Can you work these out from the model? Positions are in its coordinate system, mm. Face numbers are marked on the shaded views. A direction names the side the tool comes from. Give positions to 0.01 mm unless a question says otherwise; leave off trailing zeros. Loops run counter-clockwise (first coordinate to the right, second up) from the corner with the lowest first, then second, coordinate; pieces in that order, holes last.
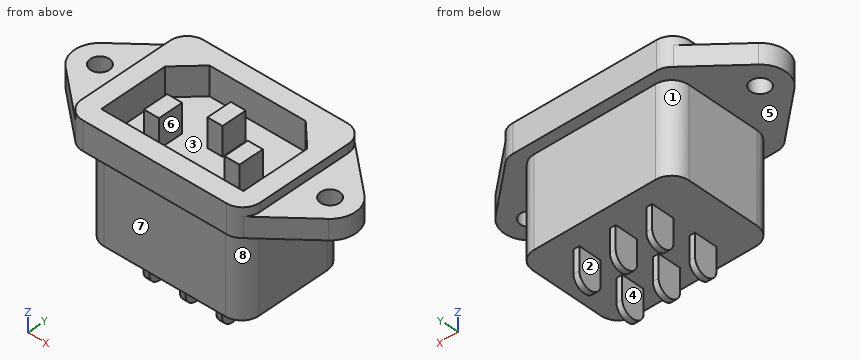
Autodesk Inventor part; units mm, degrees
ref_plane "YZ Plane" through (0, 0, 0) normal (1, 0, 0) x (0, 1, 0)
ref_plane "XZ Plane" through (0, 0, 0) normal (0, 1, 0) x (-1, 0, 0)
ref_plane "XY Plane" through (0, 0, 0) normal (0, 0, 1) x (1, 0, 0)
sketch "Base" plane through (0, 0, 0) normal (0, 0, 1) x (1, 0, 0)
  line L0 (-12.5, -11.25) -> (12.5, -11.25)
  line L1 (15.5, -8.25) -> (15.5, 8.25)
  line L2 (12.5, 11.25) -> (-12.5, 11.25)
  line L3 (-15.5, 8.25) -> (-15.5, -8.25)
  line L4 (-15.5, -11.25) -> (15.5, 11.25) construction
  line L5 (15.5, -11.25) -> (-15.5, 11.25) construction
  line L6 (-34.16, 0) -> (34.16, 0) construction
  line L7 (0, -16.6198) -> (0, 16.6198) construction
  circle A0 centre (-20, 0) radius 1.65
  circle A1 centre (20, 0) radius 1.65
  circle A2 centre (-20, 0) radius 4.4
  circle A3 centre (20, 0) radius 4.4
  line L8 (-24.4, 0) -> (24.4, 0) construction
  arc A4 (-12.5, 11.25) -> (-15.5, 8.25) centre (-12.5, 8.25) ccw
  arc A5 (-15.5, -8.25) -> (-12.5, -11.25) centre (-12.5, -8.25) ccw
  arc A6 (15.5, 8.25) -> (12.5, 11.25) centre (12.5, 8.25) ccw
  arc A7 (12.5, -11.25) -> (15.5, -8.25) centre (12.5, -8.25) ccw
  line L9 (-22.8555, 3.3476) -> (-14.6213, 10.3713)
  line L10 (14.6213, 10.3713) -> (22.8555, 3.3476)
  line L11 (-22.8555, -3.3476) -> (-14.6213, -10.3713)
  line L12 (14.6213, -10.3713) -> (22.8555, -3.3476)
  point P0 (0, 0)
  dimension "d0" = 31
  dimension "d1" = 22.5
  dimension "d2" = 3.3
  dimension "d3" = 48.8
  dimension "d4" = 40
  dimension "d15" = 3
  dimension "d16" = 3
extrude "BaseFeature" add sketch "Base" along normal blind 3.5
sketch "ReceptacleInside" plane through (0, 0, 3.5) normal (0, 0, 1) x (1, 0, 0)
  line L0 (-12.35, 7.95) -> (12.35, 7.95)
  line L1 (12.35, 7.95) -> (12.35, -7.95)
  line L2 (12.35, -7.95) -> (-12.35, -7.95)
  line L3 (-12.35, -7.95) -> (-12.35, 7.95)
  line L4 (-12.35, 7.95) -> (12.35, -7.95) construction
  line L5 (12.35, 7.95) -> (-12.35, -7.95) construction
  line L6 (-12.35, 3.95) -> (-8.35, 7.95)
  line L7 (12.35, 3.95) -> (8.35, 7.95)
  line L8 (-34.16, 0) -> (34.16, 0) construction
  line L9 (0, -15.75) -> (0, 15.75) construction
  point P0 (0, 0)
  point P1 (8.35, 7.95)
  dimension "d10" = 15.9
  dimension "d11" = 4
  dimension "d12" = 4
extrude "ReceptacleInsideFeature" cut sketch "ReceptacleInside" against normal through all contours L0 L7 L1 L2 L3 L6
sketch "Receptacle" plane through (0, 0, 3.5) normal (0, 0, 1) x (1, 0, 0)
  arc A0 (-12.5, 11.25) -> (-15.5, 8.25) centre (-12.5, 8.25) ccw
  line L0 (-15.5, 8.25) -> (-15.5, -8.25)
  arc A1 (-15.5, -8.25) -> (-12.5, -11.25) centre (-12.5, -8.25) ccw
  line L1 (-12.5, -11.25) -> (12.5, -11.25)
  arc A2 (12.5, -11.25) -> (15.5, -8.25) centre (12.5, -8.25) ccw
  line L2 (15.5, -8.25) -> (15.5, 8.25)
  arc A3 (15.5, 8.25) -> (12.5, 11.25) centre (12.5, 8.25) ccw
  line L3 (12.5, 11.25) -> (-12.5, 11.25)
  line L4 (-12.35, 3.95) -> (-8.35, 7.95)
  line L5 (-8.35, 7.95) -> (8.35, 7.95)
  line L6 (8.35, 7.95) -> (12.35, 3.95)
  line L7 (12.35, 3.95) -> (12.35, -7.95)
  line L8 (12.35, -7.95) -> (-12.35, -7.95)
  line L9 (-12.35, -7.95) -> (-12.35, 3.95)
  point P0 (0, 0)
extrude "Extrusion4" add sketch "Receptacle" along normal blind 1.5
sketch "Sketch5" plane through (0, 0, 0) normal (0, 0, -1) x (-1, 0, 0)
  line L0 (13.55, -9.35) -> (-13.55, -9.35)
  line L1 (-13.55, -9.35) -> (-13.55, 9.35)
  line L2 (-13.55, 9.35) -> (13.55, 9.35)
  line L3 (13.55, 9.35) -> (13.55, -9.35)
  line L4 (13.55, -9.35) -> (-13.55, 9.35) construction
  line L5 (-13.55, -9.35) -> (13.55, 9.35) construction
  point P0 (0, 0)
  dimension "d19" = 27.1
  dimension "d20" = 18.7
extrude "Extrusion5" add sketch "Sketch5" along normal blind 15.5
fillet "Fillet1" radius 3 4 edges at (-13.55, -9.35, -7.75) (13.55, -9.35, -7.75) (-13.55, 9.35, -7.75) (13.55, 9.35, -7.75)
sketch "Sketch6" plane through (0, 0, 0) normal (0, 0, 1) x (1, 0, 0)
  line L0 (-34.16, 0) -> (34.16, 0) construction
  line L1 (-1.3, 0) -> (1.3, 0)
  line L2 (1.3, 0) -> (1.3, 4.33)
  line L3 (1.3, 4.33) -> (-1.3, 4.33)
  line L4 (-1.3, 4.33) -> (-1.3, 0)
  line L5 (0, -15.75) -> (0, 15.75) construction
  line L6 (-8.3, 0) -> (-5.7, 0)
  line L7 (-5.7, 0) -> (-5.7, -4.33)
  line L8 (-5.7, -4.33) -> (-8.3, -4.33)
  line L9 (-8.3, -4.33) -> (-8.3, 0)
  line L10 (8.3, 0) -> (5.7, 0)
  line L11 (5.7, 0) -> (5.7, -4.33)
  line L12 (5.7, -4.33) -> (8.3, -4.33)
  line L13 (8.3, -4.33) -> (8.3, 0)
  point P0 (0, 0)
  point P1 (7, -4.33)
  point P2 (-7, -4.33)
  dimension "d24" = 14
  dimension "d25" = 2.6
  dimension "d26" = 4.33
extrude "Extrusion6" add sketch "Sketch6" along normal up to surface (5 mm away)
sketch "Sketch7" plane through (-10.55, -9.35, 0) normal (0, -1, 0) x (1, 0, 0)
  line L0 (0, -15.5) -> (21.1, -15.5)
  line L1 (3.72, -15.5) -> (4.72, -15.5)
  line L2 (4.72, -15.5) -> (4.72, -21.5)
  line L3 (4.72, -21.5) -> (3.72, -21.5)
  line L4 (3.72, -21.5) -> (3.72, -15.5)
  line L5 (10.05, -15.5) -> (11.05, -15.5)
  line L6 (11.05, -15.5) -> (11.05, -21.5)
  line L7 (11.05, -21.5) -> (10.05, -21.5)
  line L8 (10.05, -21.5) -> (10.05, -15.5)
  line L9 (16.38, -15.5) -> (17.38, -15.5)
  line L10 (17.38, -15.5) -> (17.38, -21.5)
  line L11 (17.38, -21.5) -> (16.38, -21.5)
  line L12 (16.38, -21.5) -> (16.38, -15.5)
  line L13 (10.55, -21.5) -> (10.55, 5) construction
  line L14 (11.85, 5) -> (9.25, 5)
  line L15 (10.55, -26.8) -> (10.55, 10.3) construction
  point P0 (10.55, 0)
  point P1 (4.72, -15.5)
  dimension "d29" = 6
  dimension "d30" = 5.33
  dimension "d31" = 5.33
  dimension "d32" = 1
extrude "Extrusion7" add sketch "Sketch7" against normal up to surface (18.7 mm away)
sketch "Sketch8" plane through (6.83, -9.35, -15.5) normal (1, 0, 0) x (0, 0, -1)
  circle A0 centre (4, 5.35) radius 2
  line L0 (6, 0) -> (6, 18.7)
  line L1 (0, 0) -> (0, 18.7)
  line L2 (4, 3.35) -> (0, 3.35)
  line L3 (0, 3.35) -> (0, 7.35)
  line L4 (0, 7.35) -> (4, 7.35)
  line L5 (4, 7.35) -> (4, 3.35)
  line L6 (11.3, 9.35) -> (-25.8, 9.35) construction
  circle A1 centre (4, 13.35) radius 2
  line L7 (4, 15.35) -> (0, 15.35)
  line L8 (0, 11.35) -> (4, 11.35)
  line L9 (6, 18.7) -> (0, 18.7)
  line L10 (0, 0) -> (0, 18.7)
  line L11 (6, 0) -> (0, 0)
  line L12 (6, 0) -> (6, 18.7)
  point P0 (-15.5, 9.35)
  point P1 (6, 5.35)
  point P2 (0, 3.35)
  point P3 (6, 13.35)
  point P4 (0, 15.35)
  dimension "d35" = 4
  dimension "d36" = 4
  dimension "d37" = 4
  dimension "d38" = 2
extrude "Extrusion8" cut sketch "Sketch8" against normal through all contours L0 L11 L1 L2 A0 | A0 L4 L1 L8 A1 L0 | A1 L7 L1 L9 L0
equation "\"d27\" = d25"
equation "\"d33\" = d30"
properties part number "Qteatak"
(1) Suppose I cut it at B-B on x = 5. List the corners of the cut face in (y, z) for me, plus the area to 3 significant figures.
Returned:
outline: (-11.25, 0) - (-9.35, 0) - (-9.35, -15.5) - (9.35, -15.5) - (9.35, 0) - (11.25, 0) - (11.25, 5) - (7.95, 5) - (7.95, 0) - (-7.95, 0) - (-7.95, 5) - (-11.25, 5) - close
area: 323 mm2
(2) Suppose I cut it at A-A on z = -18. List the corners of the cut face in (x, y) for me.
Returned:
outline: (-6.83, -6) - (-5.83, -6) - (-5.83, -2) - (-6.83, -2) - close; (-6.83, 2) - (-5.83, 2) - (-5.83, 6) - (-6.83, 6) - close; (-0.5, -6) - (0.5, -6) - (0.5, -2) - (-0.5, -2) - close; (-0.5, 2) - (0.5, 2) - (0.5, 6) - (-0.5, 6) - close; (5.83, -6) - (6.83, -6) - (6.83, -2) - (5.83, -2) - close; (5.83, 2) - (6.83, 2) - (6.83, 6) - (5.83, 6) - close
(3) Which directions (+Z, -Z, +X, -X, +Y, -Y) give clear straight access to the entire face, cutting with the end or side of a thin tool? Please do the marked faces 4, 5, 6, 7 and 8.
Returned:
face 4: -Z, +Y, -Y
face 5: -Z
face 6: +Z
face 7: -Z, +X, -X, -Y
face 8: -Z, +X, -Y
(4) Thinking about a two-plate mould opening in Y: for the marked faces 1, 2 and 3, which applies, pulls with the +Y half, pulls with the -Y half, needs draft (parallel to the pull), parting line crosses it, or undercut?
Returned:
face 1: pulls with the +Y half
face 2: needs draft
face 3: undercut
(5) Please list where these lines run through material, in increasing order: probe 1 along X at (y, z) = (3.5, 3); probe 2 along Z at (x, y) = (10.5, 9.5); probe 3 along Z at (x, y) = (21, -3).
Returned:
probe 1: x = -22.68 to -12.35, -1.3 to 1.3, 12.35 to 22.68
probe 2: z = 0 to 5
probe 3: z = 0 to 3.5
(6) Suppose I cut it at C-C on z = 2.75. Give the number of separate pieces and of enclosed holes in the cut face, plus the area to 3 significant figures.
Returned:
separate pieces: 4
enclosed holes: 3
area: 536 mm2
(7) Suppose I cut it at D-D on x = -20. List the corners of the cut face in (y, z) for me.
Returned:
outline: (-5.78, 0) - (-1.65, 0) - (-1.65, 3.5) - (-5.78, 3.5) - close; (1.65, 0) - (5.78, 0) - (5.78, 3.5) - (1.65, 3.5) - close
(8) Will these pins go through, and if not, where does the flat tip stop? P1, Ø5, axis at y = 0, z = -17, coming from the +X side; P2, Ø0.8, axis at x = -6, z = -17.5, coming from the -Y side; P3, Ø4.5, axis at y = 4.5, z = -17.5, coming from the -X side; P4, Ø1, axis at x = -3.5, z = -16.5, coming from the -Y side.
Returned:
P1: stops at x = 13.55
P2: stops at y = -6
P3: stops at x = -13.55
P4: passes through
